Design review of the part built by this model. Coordinates are the model's own, in mm. A direction names the side the tool comes from. Give positions to 0.01 mm unless a question says otherwise; leave off trailing zeros. Loops run counter-clockwise (first coordinate to the right, second up) from the corner with the lowest first, then second, coordinate; pieces in that order, holes last. Notation, with made-up numbers: (59, 26.25) -> (89, 26.25) arc R21 cw to (89, 55.25) -> close; hole circle Ø8 at (29, 77.5). An arc over 180 degrees is marked (long way). Answer in a Markdown table with one row per item. Add a question column.
(1) Consider section A-A on x = 45.5. Count the separate pieces of the cut face and the enclosed holes in it, then the cut area to 3 significant figures.
(2) For line 1 (Z direction, x = 14.5, y = 73.85); line 2 (Z direction, x = 30, y = 1); line 3 (Y direction, x = 38, z = -30.5), list the stretches that pass through material, from the lowest coordinate up.
(3) Consider section C-C on x = 22.5. Write out the cut boundary in (y, z).
(4) Draft analysis for pull direction Z (two halves, no side actions). For faces 3 (the cylindrical face through (44.036, 2.465, -5.925)), 4 (the flat face through (35, 70, -21)), 5 (the flat face through (5, 38, -37)), state which applies: +Z half, -Z half, draft (parallel to the pull), parting line (faces both ways), or undercut.
(5) For faces 1 (the flat face through (35, 5, -21)), 2 (the flat face through (30, 75, -17)), list the 3-axis set-ups (+Z, -Z, +X, -X, +Y, -Y) from which the entire face can be reached by the end or side of a thin tool; tool diameter is ignored.
from build123d import *

# Parameters (mm, degrees)
SKETCH3_W           = 60
SKETCH3_H           = 42
SKETCH3_R           = 3.75
SKETCH3_R_2         = 1.5
BOSS_EXTRUDE1_DEPTH = 75
SKETCH4_W           = 60
SKETCH4_H           = 65
CUT_EXTRUDE1_DEPTH  = 105.828431258
BOSS_EXTRUDE2_REACH = 103.311
SKETCH5_W           = 10
SKETCH5_H           = 42
CHAMFER2_SIZE       = 10


with BuildPart() as part:
    # Sketch3 → Boss-Extrude1 (new body)
    with BuildSketch(Plane(origin=(0, 0, 0), x_dir=(1, 0, 0), z_dir=(0, 1, 0))):
        with Locations((30, 21)):
            Rectangle(SKETCH3_W, SKETCH3_H)
        with Locations(Location((30, 21, 0), (0, 0, 270))):
            Circle(SKETCH3_R, mode=Mode.SUBTRACT)
        with Locations(Location((14.5, 36.4, 0), (0, 0, 270))):
            Circle(SKETCH3_R_2, mode=Mode.SUBTRACT)
        with Locations(Location((45.5, 36.4, 0), (0, 0, 270))):
            Circle(SKETCH3_R_2, mode=Mode.SUBTRACT)
        with Locations(Location((45.5, 5.6, 0), (0, 0, 270))):
            Circle(SKETCH3_R_2, mode=Mode.SUBTRACT)
        with Locations(Location((14.5, 5.6, 0), (0, 0, 270))):
            Circle(SKETCH3_R_2, mode=Mode.SUBTRACT)
        with Locations(Location((30, 36.4, 0), (0, 0, 270))):
            Circle(SKETCH3_R_2, mode=Mode.SUBTRACT)
        with Locations(Location((45.5, 21, 0), (0, 0, 270))):
            Circle(SKETCH3_R_2, mode=Mode.SUBTRACT)
        with Locations(Location((30, 5.6, 0), (0, 0, 270))):
            Circle(SKETCH3_R_2, mode=Mode.SUBTRACT)
        with Locations(Location((14.5, 21, 0), (0, 0, 270))):
            Circle(SKETCH3_R_2, mode=Mode.SUBTRACT)
    extrude(amount=BOSS_EXTRUDE1_DEPTH)

    # Sketch4 → Cut-Extrude1 (cut, through all)
    with BuildSketch(Plane(origin=(0, 0, -42), x_dir=(-1, 0, 0), z_dir=(0, 0, -1))):
        with Locations((-30, 37.5)):
            Rectangle(SKETCH4_W, SKETCH4_H)
    extrude(amount=-CUT_EXTRUDE1_DEPTH, mode=Mode.SUBTRACT)


with BuildPart() as cut_extrude1_piece_1:
    # of the separate pieces the step leaves, piece 1, a body of its own (cut_extrude1_pieces)
    add(part.part.solids().sort_by_distance((60, 70, 0))[0])

    # Sketch5 → Boss-Extrude2 (add, up to next)
    with BuildSketch(Plane(origin=(0, 5, 0), x_dir=(1, 0, 0), z_dir=(0, 1, 0)), mode=Mode.PRIVATE) as boss_extrude2_sk1:
        with Locations((5, 21)):
            Rectangle(SKETCH5_W, SKETCH5_H)
    boss_extrude2_tool1 = extrude(boss_extrude2_sk1.sketch, amount=BOSS_EXTRUDE2_REACH, mode=Mode.PRIVATE) - cut_extrude1_piece_1.part
    # Sketch5 → Boss-Extrude2 (add, up to next)
    with BuildSketch(Plane(origin=(0, 5, 0), x_dir=(1, 0, 0), z_dir=(0, 1, 0)), mode=Mode.PRIVATE) as boss_extrude2_sk2:
        with Locations((55, 21)):
            Rectangle(SKETCH5_W, SKETCH5_H)
    boss_extrude2_tool2 = extrude(boss_extrude2_sk2.sketch, amount=BOSS_EXTRUDE2_REACH, mode=Mode.PRIVATE) - cut_extrude1_piece_1.part


with BuildPart() as cut_extrude1_piece_2:
    # of the separate pieces the step leaves, piece 2, a body of its own (cut_extrude1_pieces)
    add(part.part.solids().sort_by_distance((0, 0, 0))[0])


with BuildPart() as cut_extrude1_piece_1_1:
    add(cut_extrude1_piece_1.part)

    add(cut_extrude1_piece_2.part)  # Boss-Extrude2 merges Cut-Extrude1 piece 2
    add(boss_extrude2_tool1.solids().sort_by_distance((5, 5, -21))[0])
    add(boss_extrude2_tool2.solids().sort_by_distance((55, 5, -21))[0])

    # Chamfer2
    chamfer2_edges = [cut_extrude1_piece_1_1.edges().sort_by_distance(p)[0] for p in [
        (0, 37.5, -42),
        (0, 37.5, 0),
        (60, 37.5, 0),
        (60, 37.5, -42),
    ]]
    chamfer(chamfer2_edges, length=CHAMFER2_SIZE - 0.0001)  # a hair under: the kernel refuses the full size


solid = cut_extrude1_piece_1_1.part
Values follow:
| question | item | result |
|---|---|---|
| 1 | separate pieces | 8 |
| 1 | enclosed holes | 0 |
| 1 | area | 330 mm2 |
| 2 | line 1 | -42 to -37.9, -34.9 to -22.5, -19.5 to -7.1, -4.1 to 0 |
| 2 | line 2 | -42 to -37.9, -34.9 to -24.75, -17.25 to -7.1, -4.1 to 0 |
| 2 | line 3 | 0 to 5, 70 to 75 |
| 3 | outline | (0, -42) -> (5, -42) -> (5, 0) -> (0, 0) -> close; (70, -42) -> (75, -42) -> (75, 0) -> (70, 0) -> close |
| 4 | face 3 | undercut |
| 4 | face 4 | draft |
| 4 | face 5 | -Z half |
| 5 | face 1 | +Z, -Z |
| 5 | face 2 | +Z, -Z, +X, -X, +Y |
